Geometry: final body of the model. Coordinates: model frame, mm. Give positions to 0.01 mm unless a question says otherwise; leave off trailing zeros. Loops run counter-clockwise (first coordinate to the right, second up) from the corner with the lowest first, then second, coordinate; pieces in that order, holes last.
from build123d import *

# Parameters (mm, degrees)
F0_W     = 92.25
F0_H     = 92.25
F1_DEPTH = 25
F2_R     = 43.5
F3_DEPTH = 25.001
F5_D     = 4.3
F6_R     = 3


with BuildPart() as f1:
    # F0 (on Front) → F1 (new body)
    with BuildSketch(Plane.XZ):
        with Locations((46.125, 46.125)):
            Rectangle(F0_W, F0_H)
    extrude(amount=F1_DEPTH)

    # F2 (on face) → F3 (cut, through all)
    with BuildSketch(Plane.XZ.offset(25)):
        with Locations((46.125, 46.125)):
            Circle(F2_R)
    extrude(amount=-F3_DEPTH, mode=Mode.SUBTRACT)

    # F5 (through all)
    with Locations(Plane.XZ.offset(25)):
        with Locations((5.3, 86.95), (5.3, 5.3), (86.95, 5.3), (86.95, 86.95)):
            Hole(F5_D / 2)

    # F6
    f6_edges = [f1.edges().sort_by_distance(p)[0] for p in [
        (92.25, -12.5, 92.25),
        (0, -12.5, 92.25),
        (0, -12.5, 0),
        (92.25, -12.5, 0),
    ]]
    fillet(f6_edges, radius=F6_R)


solid = f1.part
Item 1: Ray query, probe 1 along X at (y, z) = (-8, 45.5); probe 2 along Z at (x, y) = (52, -10.5). Return the intervals inside material, ascending.
Values follow:
probe 1: x = 0 to 2.63, 89.62 to 92.25
probe 2: z = 0 to 3.02, 89.23 to 92.25
Item 2: Section query D-D on x = 5.3. Return loops of the section in (y, z), plus the area to 3 significant figures.
Values follow:
outline: (-25, 0) - (0, 0) - (0, 3.15) - (-25, 3.15) - close; (-25, 7.45) - (0, 7.45) - (0, 31.11) - (-25, 31.11) - close; (-25, 61.14) - (0, 61.14) - (0, 84.8) - (-25, 84.8) - close; (-25, 89.1) - (0, 89.1) - (0, 92.25) - (-25, 92.25) - close
area: 1,340 mm2
Item 3: Draft query along Z for faces 1 (the face through (4.14, -12.32, 7.11)), 2 (the face through (46, -12, 0)), 3 (the face through (11.7, 0, 19)). Return one class per face: +Z half, -Z half, draft (parallel to the pull), parting line (faces both ways), or undercut.
Values follow:
face 1: undercut
face 2: -Z half
face 3: draft
Item 4: Section query B-B on x = 77.5. Return loops of the section in (y, z).
Values follow:
outline: (-25, 0) - (0, 0) - (0, 15.99) - (-25, 15.99) - close; (-25, 76.26) - (0, 76.26) - (0, 92.25) - (-25, 92.25) - close
Item 5: Section query A-A on z = 48. Return loops of the section in (x, y), plus the area to 3 significant figures.
Values follow:
outline: (0, -25) - (2.67, -25) - (2.67, 0) - (0, 0) - close; (89.58, -25) - (92.25, -25) - (92.25, 0) - (89.58, 0) - close
area: 133 mm2
Item 6: Section query C-C on y = -4.5. Return loops of the section in (x, z) (3 decimals), plus the area to 3 significant figures.
Values follow:
outline: (0, 3) arc R3 ccw to (3, 0) - (89.25, 0) arc R3 ccw to (92.25, 3) - (92.25, 89.25) arc R3 ccw to (89.25, 92.25) - (3, 92.25) arc R3 ccw to (0, 89.25) - close; hole circle Ø87 at (46.125, 46.125); hole circle Ø4.3 at (5.3, 5.3); hole circle Ø4.3 at (5.3, 86.95); hole circle Ø4.3 at (86.95, 5.3); hole circle Ø4.3 at (86.95, 86.95)
area: 2,500 mm2
